Can you work these out from the model? Positions are in its coordinate system, mm. Face numbers are marked on the shaded views. A direction names the side the tool comes from. Give positions to 0.01 mm unless a question says otherwise; leave off trailing zeros. Order: outer loops, then holes, each group sorted by start corner. A loop starts at its lowest first (then second) coordinate and runs counter-clockwise, first axis right, second up. Notation, with made-up numbers: (77.25, -25) - (133.25, -25) arc R21 cw to (133.25, 7) - close; hole circle Ø6 at (60, 2.5). An arc over 180 degrees is marked (long way). One line per question, with ' | ' between items.
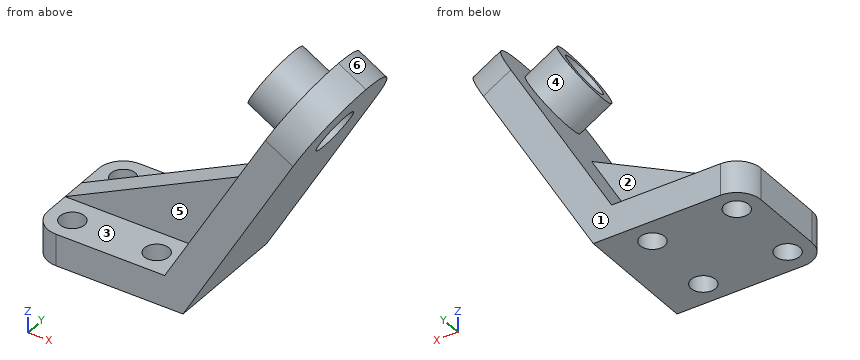
```python
from build123d import *

# Parameters (mm, degrees)
F1_DEPTH  = 102
F2_R      = 50.99999
F3_R      = 27
F3_R_2    = 18.5
F4_DEPTH  = 30
F5_R      = 18.5
F6_DEPTH  = 30
F9_DEPTH  = 10
F10_R     = 10
F11_DEPTH = 30
F12_R     = 20


# Not quite as in the source:
# - a fillet or chamfer is up to 0.001 mm smaller than in the source, because OpenCascade refuses the exact size


with BuildPart() as f1:
    # F0 (on Front) → F1 (new body)
    with BuildSketch(Plane.XZ):
        Polygon((-15.0111069989, -63.9414438152), (-124.0111069989, -63.9414438152), (-124.0111069989, -89.9414438152), (0, -89.9414438152), (115.5, 110.110424459), (92.9833395016, 123.110424459), align=None)
    extrude(amount=F1_DEPTH)

    # F2 (radius 51 in the source; OpenCascade refuses exactly that, so slightly less here)
    f2_edges = [f1.edges().sort_by_distance(p)[0] for p in [
        (104.24167, 0, 116.610424),
        (104.24167, -102, 116.610424),
    ]]
    fillet(f2_edges, radius=F2_R)

    # F3 (on face) → F4 (join)
    with BuildSketch(Plane(origin=(16.4291271001, 0, -9.4853609538), x_dir=(0, -1, 0), z_dir=(-0.8660254038, 0, 0.5))):
        with Locations((51, 102.108424803)):
            Circle(F3_R)
        with Locations((51, 102.108424803)):
            Circle(F3_R_2, mode=Mode.SUBTRACT)
    extrude(amount=F4_DEPTH)

    # F5 (on face) → F6 (cut)
    with BuildSketch(Plane(origin=(16.4291271001, 0, -9.4853609538), x_dir=(0, -1, 0), z_dir=(-0.8660254038, 0, 0.5))):
        with Locations((51, 102.108424803)):
            Circle(F5_R)
    extrude(amount=-F6_DEPTH, mode=Mode.SUBTRACT)

    # F8 (on offset) → F9 (join, symmetric)
    with BuildSketch(Plane(origin=(0, -51, 0), x_dir=(-1, 0, 0), z_dir=(0, 1, 0))):
        Polygon((-28.8675134595, 12.0585561848), (15.0111069989, -63.9414438152), (124.0111069989, -63.9414438152), align=None)
    extrude(amount=F9_DEPTH, both=True)

    # F10 (on face) → F11 (cut)
    with BuildSketch(Plane.XY.offset(-63.9414438152)):
        with Locations((-104.0111069989, -20)):
            Circle(F10_R)
        with Locations((-104.0111069989, -82)):
            Circle(F10_R)
        with Locations((-35.0111069989, -20)):
            Circle(F10_R)
        with Locations((-35.0111069989, -82)):
            Circle(F10_R)
    extrude(amount=-F11_DEPTH, mode=Mode.SUBTRACT)

    # F12
    f12_edges = [f1.edges().sort_by_distance(p)[0] for p in [
        (-124.011107, 0, -76.941444),
        (-124.011107, -102, -76.941444),
    ]]
    fillet(f12_edges, radius=F12_R)


solid = f1.part
```
(1) Imagine slicing it at B-B (z = -28). List the corners of the cut face in (x, y) for me.
Answer below:
outline: (-51.71, -61) - (5.74, -61) - (5.74, -102) - (35.76, -102) - (35.76, 0) - (5.74, 0) - (5.74, -41) - (-51.71, -41) - close
(2) If I drill on line 1 (X direction, y = -19, z = -67.5); line 2 (Y direction, x = -59, z = -32.5); line 3 (Z direction, x = -77.5, y = -36), over which ranges is the centre line in solid material (lowest first)?
Answer below:
line 1: -123.99 to -113.96, -94.06 to -44.96, -25.06 to 12.96 | line 2: -61 to -41 | line 3: -89.94 to -63.94
(3) Will these pins go through, and if not, where does the flat tip stop? pin 1 (10 mm diameter, centred on x = 25, z = 7, fed in from +Y); pin 2 (1.5 mm diameter, centred on x = -49.5, y = -52.5, fed in from +Z); pin 3 (1 mm diameter, centred on x = 86, y = -63.5, fed in from -Z); pin 4 (12.5 mm diameter, centred on x = -54, y = -24.5, fed in from +Z).
Answer below:
pin 1: y = 0 | pin 2: z = -26.53 | pin 3: z = 83.38 | pin 4: z = -63.94
(4) Imagine slicing it at A-A (x = -72.5). List the corners of the cut face in (y, z) for me, and give its area (3 significant figures).
Answer below:
outline: (-102, -89.94) - (0, -89.94) - (0, -63.94) - (-41, -63.94) - (-41, -38.33) - (-61, -38.33) - (-61, -63.94) - (-102, -63.94) - close | area: 3,160 mm^2
(5) If we mould it in two halves opening along Z, with no side actions, what happens to the marked faces 4, 5 and 6? For each: released by +Z, released by -Z, zero draft, split by the parting line, or undercut.
Answer below:
face 4: undercut | face 5: zero draft | face 6: released by +Z
(6) On a 3-axis mill with a long thin cutter (end or side, diameter ignored), from which of +Z, -Z, +X, -X, +Y, -Y can I reach the whole of each face in a straight line? I mean the marked faces 1, 2 and 3. Say none if no direction works.
Answer below:
face 1: +Z, -Z, +X, -X, +Y | face 2: +Z, -X, +Y | face 3: +Z, -X, -Y
